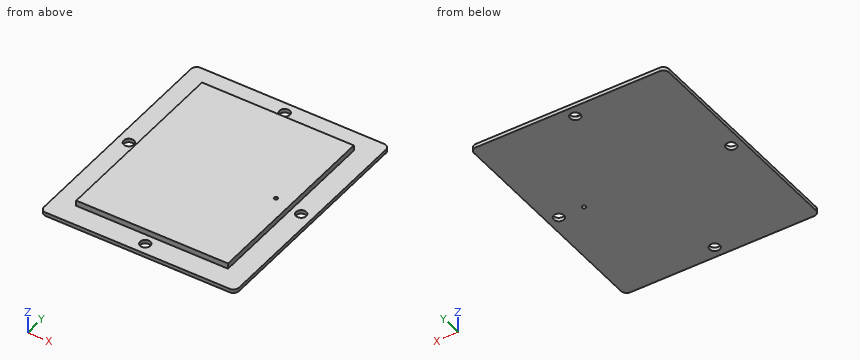
from build123d import *

# Parameters (mm, degrees)
SKETCH1_W           = 104
SKETCH1_H           = 124
BOSS_EXTRUDE1_DEPTH = 2
SKETCH4_W           = 81
SKETCH4_H           = 101
BOSS_EXTRUDE2_DEPTH = 3
SKETCH5_R           = 1
CUT_EXTRUDE1_DEPTH  = 162.916645222
FILLET1_R           = 3
SKETCH6_R           = 2.75
CUT_EXTRUDE3_DEPTH  = 162.867229543
SKETCH9_R           = 2.75
CUT_EXTRUDE4_DEPTH  = 162.867229543


with BuildPart() as part:
    # Sketch1 → Boss-Extrude1 (new body)
    with BuildSketch(Plane.XY):
        with Locations((52, 62)):
            Rectangle(SKETCH1_W, SKETCH1_H)
    extrude(amount=BOSS_EXTRUDE1_DEPTH)

    # Sketch4 → Boss-Extrude2 (add)
    with BuildSketch(Plane.XY.offset(2)):
        with Locations((52, 62)):
            Rectangle(SKETCH4_W, SKETCH4_H)
    extrude(amount=BOSS_EXTRUDE2_DEPTH)

    # Sketch5 → Cut-Extrude1 (cut, through all)
    with BuildSketch(Plane.XY.offset(5)):
        with Locations((84.533228661, 62)):
            Circle(SKETCH5_R)
    extrude(amount=-CUT_EXTRUDE1_DEPTH, mode=Mode.SUBTRACT)

    # Fillet1
    fillet1_edges = [part.edges().sort_by_distance(p)[0] for p in [
        (0, 0, 1),
        (104, 0, 1),
        (104, 124, 1),
        (0, 124, 1),
    ]]
    fillet(fillet1_edges, radius=FILLET1_R)

    # Sketch6 → Cut-Extrude3 (cut, through all)
    with BuildSketch(Plane.XY.offset(2)):
        with Locations((98, 62)):
            Circle(SKETCH6_R)
        with Locations((6, 62)):
            Circle(SKETCH6_R)
    extrude(amount=-CUT_EXTRUDE3_DEPTH, mode=Mode.SUBTRACT)

    # Sketch9 → Cut-Extrude4 (cut, through all)
    with BuildSketch(Plane.XY.offset(2)):
        with Locations((52, 6)):
            Circle(SKETCH9_R)
        with Locations((52, 118)):
            Circle(SKETCH9_R)
    extrude(amount=-CUT_EXTRUDE4_DEPTH, mode=Mode.SUBTRACT)


solid = part.part
Could you check a few things on this model? Use its own coordinates, in mm. Give positions to 0.01 mm unless a question says otherwise; leave off trailing zeros. Order: outer loops, then holes, each group sorted by start corner. A loop starts at its lowest first (then second) coordinate and runs counter-clockwise, first axis right, second up.
Item 1: If we section it at D-D, the plane z = 3.7: Write out the boundary of the cut face in (x, y), plus the area to 3 significant figures.
Item 2: I'm going to push flat-ended pins straight in: pin 1 (4.5 mm diameter, centred on x = 52, y = 6, fed in from +Z); pin 2 (2.5 mm diameter, centred on y = 59, z = 4, fed in from -X); pin 3 (2.5 mm diameter, centred on x = 38, z = 3.5, fed in from +Y); pin 4 (7 mm diameter, centred on x = 52, y = 118, fed in from +Z). Where does each tip first touch, or does it pass through?
Item 3: I need wall thicknesses on line 1 (Y direction, x = 52, z = 1.2); line 2 (Y direction, x = 25.5, z = 4.25); line 3 (X direction, y = 101, z = 3.85). Which ranges of each line are inside material? Lowest first, please.
Item 4: If we section it at B-B, the plane x = 52: Write out the boundary of the cut face in (y, z), plus the area to 3 significant figures.
Item 5: If we section it at A-A, the plane y = 118: Write out the boundary of the cut face in (x, z), plus the area to 3 significant figures.
Item 6: If we section it at C-C, the plane x = 98: Write out the boundary of the cut face in (y, z), plus the area to 3 significant figures.
Values:
1. outline: (11.5, 11.5) - (92.5, 11.5) - (92.5, 112.5) - (11.5, 112.5) - close; hole circle Ø2 at (84.53, 62)
1. area: 8,180 mm2
2. pin 1: passes through
2. pin 2: stops at x = 11.5
2. pin 3: stops at y = 112.5
2. pin 4: stops at z = 2
3. line 1: y = 0 to 3.25, 8.75 to 115.25, 120.75 to 124
3. line 2: y = 11.5 to 112.5
3. line 3: x = 11.5 to 92.5
4. outline: (0, 0) - (3.25, 0) - (3.25, 2) - (0, 2) - close; (8.75, 0) - (115.25, 0) - (115.25, 2) - (112.5, 2) - (112.5, 5) - (11.5, 5) - (11.5, 2) - (8.75, 2) - close; (120.75, 0) - (124, 0) - (124, 2) - (120.75, 2) - close
4. area: 529 mm2
5. outline: (0, 0) - (49.25, 0) - (49.25, 2) - (0, 2) - close; (54.75, 0) - (104, 0) - (104, 2) - (54.75, 2) - close
5. area: 197 mm2
6. outline: (0, 0) - (59.25, 0) - (59.25, 2) - (0, 2) - close; (64.75, 0) - (124, 0) - (124, 2) - (64.75, 2) - close
6. area: 237 mm2
